Check sheet for the modelled part. Datum: model origin and axes. Units: mm. Face numbers are marked on the shaded views. Round coordinates to 2 decimals unless told otherwise and drop trailing zeros. Write each loop counter-clockwise with the first axis right and the second up, starting at its lowest first coordinate (ties: lowest second). Pieces come first, ordered by that corner, then holes.
Item 1: Section check D-D, the plane z = 5.5. Record the cut outline in (x, y).
Item 2: Section check B-B, the plane x = 0.3. Record the cut outline in (y, z), plus the area to 3 significant figures.
Item 3: Section check A-A, the plane y = 0. Record the cut outline in (x, z).
Item 4: Section check C-C, the plane z = 8. Record the cut outline in (x, y).
Item 5: Depth check by flat-ended pin: pin 1 (2 mm diameter, centred on y = 1.5, z = 2, fed in from -X); pin 2 (1.8 mm diameter, centred on x = 0, y = 0, fed in from +Z). Enter the tip coordinate at first touch or a pass-through.
Item 6: Material ranges on line 1 along Z through (x, y) = (-0.15, 1.55); line 2 along Z through (x, y) = (0.55, -0.65); line 3 along Y through (x, z) = (0.3, 11.25), recorded low to high.
Item 7: Release check for a two-part mould opening along Y. For the marked faces 1, 2, 3 and 4 record: pulls with the +Y half, pulls with the -Y half, needs draft (parallel to the pull), parting line crosses it, or undercut.
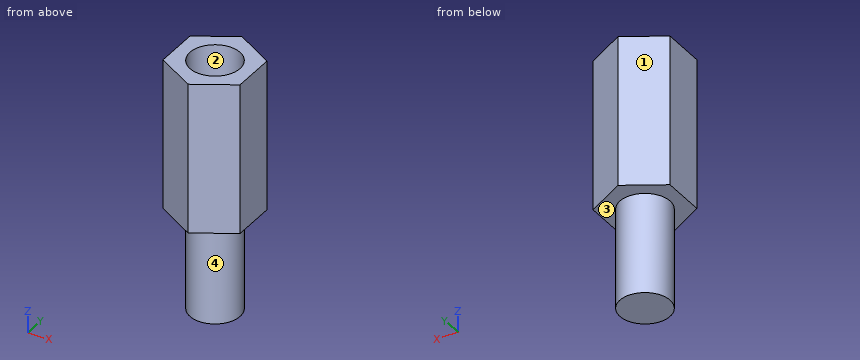
Autodesk Inventor part; units mm, degrees
ref_plane "YZ Plane" through (0, 0, 0) normal (1, 0, 0) x (0, 1, 0)
ref_plane "XZ Plane" through (0, 0, 0) normal (0, 1, 0) x (-1, 0, 0)
ref_plane "XY Plane" through (0, 0, 0) normal (0, 0, 1) x (1, 0, 0)
sketch "Sketch6" plane through (0, 0, 0) normal (0, 0, 1) x (1, 0, 0)
  line L0 (0, 2.6558) -> (2.3, 1.3279)
  line L1 (2.3, 1.3279) -> (2.3, -1.3279)
  line L2 (2.3, -1.3279) -> (0, -2.6558)
  line L3 (0, -2.6558) -> (-2.3, -1.3279)
  line L4 (-2.3, -1.3279) -> (-2.3, 1.3279)
  line L5 (-2.3, 1.3279) -> (0, 2.6558)
  point P0 (0, 0)
  point P1 (0, 0)
  dimension "d15" = 4.6
extrude "Extrusion3" add sketch "Sketch6" along normal blind 15
sketch "Sketch7" plane through (0, 0, 0) normal (0, 0, -1) x (-1, 0, 0)
  circle A0 centre (0, 0) radius 1.5
  line L0 (0, 2.6558) -> (2.3, 1.3279)
  line L1 (0, 2.6558) -> (2.3, 1.3279)
  line L2 (2.3, 1.3279) -> (2.3, -1.3279)
  line L3 (2.3, -1.3279) -> (0, -2.6558)
  line L4 (0, -2.6558) -> (-2.3, -1.3279)
  line L5 (-2.3, -1.3279) -> (-2.3, 1.3279)
  line L6 (-2.3, 1.3279) -> (0, 2.6558)
  dimension "d18" = 3
extrude "Extrusion4" cut sketch "Sketch7" against normal blind 6
thread "Thread2"
sketch "Sketch8" plane through (0, 0, 15) normal (0, 0, 1) x (1, 0, 0)
  circle A0 centre (0, 0) radius 1.5
  dimension "d23" = 3
extrude "Extrusion5" cut sketch "Sketch8" against normal blind 6
thread "Thread3"
equation "\"BendRadius\" = Thickness"
equation "\"BendReliefWidth\" = Thickness"
equation "\"BendReliefDepth\" = 0.5 * Thickness"
equation "\"CornerReliefSize\" = 4 * Thickness"
equation "\"MinimumRemnant\" = 2 * Thickness"
equation "\"TransitionRadius\" = BendRadius"
equation "\"JacobiRadiusSize\" = Thickness"
equation "\"GapSize\" = Thickness"
properties part number "PCB SEPARADOR" material "Stainless Steel"
Values found:
1. outline: circle Ø3 at (0, 0)
2. outline: (-2.48, 6) - (-1.47, 6) - (-1.47, 0) - (1.47, 0) - (1.47, 6) - (2.48, 6) - (2.48, 15) - (1.47, 15) - (1.47, 9) - (-1.47, 9) - (-1.47, 15) - (-2.48, 15) - close
2. area: 44.7 mm2
3. outline: (-2.3, 6) - (-1.5, 6) - (-1.5, 0) - (1.5, 0) - (1.5, 6) - (2.3, 6) - (2.3, 15) - (1.5, 15) - (1.5, 9) - (-1.5, 9) - (-1.5, 15) - (-2.3, 15) - close
4. outline: (-2.3, -1.33) - (0, -2.66) - (2.3, -1.33) - (2.3, 1.33) - (0, 2.66) - (-2.3, 1.33) - close
5. pin 1: stops at x = -1.41
5. pin 2: stops at z = 9
6. line 1: z = 6 to 15
6. line 2: z = 0 to 9
6. line 3: y = -2.48 to -1.47, 1.47 to 2.48
7. face 1: pulls with the +Y half
7. face 2: undercut
7. face 3: needs draft
7. face 4: parting line crosses it
